CAD build for the part. Positions are in the model's coordinates, mm. A direction names the side the tool comes from. Coordinates: 2 decimals unless noted, no trailing zeros. Write each loop counter-clockwise with the first axis right and the second up, starting at its lowest first coordinate (ties: lowest second). Pieces come first, ordered by that corner, then holes.
```python
from build123d import *

# Parameters (mm, degrees)
SKETCH1_W              = 42
SKETCH1_H              = 5.9
SKETCH1_W_2            = 39.2
SKETCH1_H_2            = 3.95
BOSS_EXTRUDE1_DEPTH    = 32.25
FILLET2_R              = 3
SKETCH2_W              = 51.5
SKETCH2_H              = 13.6
SKETCH2_W_2            = 39.2
SKETCH2_H_2            = 3.95
BOSS_EXTRUDE2_DEPTH    = 5.8
SKETCH3_W              = 51.5
SKETCH3_H              = 13.6
SKETCH3_W_2            = 39.2
SKETCH3_H_2            = 3.95
BOSS_EXTRUDE3_DEPTH    = 5.8
SKETCH4_R              = 1.7
CUT_EXTRUDE1_DEPTH     = 62.792596644
SKETCH8_W              = 5.8
SKETCH8_H              = 7.5
BOSS_EXTRUDE4_DEPTH    = 13.6
M2_CLEARANCE_HOLE1_D   = 2.4
CUT_EXTRUDE4_DEPTH     = 4
SKETCH15_W             = 39.2
SKETCH15_H             = 3.95
CUT_EXTRUDE5_DEPTH     = 79.468767672
SKETCH17_R             = 2
CUT_EXTRUDE6_DEPTH     = 79.468767672
M3_CLEARANCE_HOLE1_D   = 3.4
CUT_EXTRUDE8_START     = -13.6
CUT_EXTRUDE8_OUTLINE_W = 5.8
CUT_EXTRUDE8_OUTLINE_H = 7.5
CUT_EXTRUDE8_OUTLINE_R = 1.7
CUT_EXTRUDE8_DEPTH     = 4.55
FILLET3_R              = 1


# Read off the part's stored shape, not the designer's step: Cut-Extrude8
with BuildPart() as part:
    # Sketch1 → Boss-Extrude1 (new body)
    with BuildSketch(Plane(origin=(0, 0, 0), x_dir=(0, 0, -1), z_dir=(1, 0, 0))):
        with Locations((21, 2.95)):
            Rectangle(SKETCH1_W, SKETCH1_H)
        with Locations((21, 2.95)):
            Rectangle(SKETCH1_W_2, SKETCH1_H_2, mode=Mode.SUBTRACT)
    extrude(amount=BOSS_EXTRUDE1_DEPTH)

    # Fillet2
    # the kernel refuses this fillet: 3 mm, written as the material it takes off along each edge
    with BuildSketch(Plane(origin=(-7.5, 0, -42), x_dir=(0, 0, 1), z_dir=(1, 0, 0)), Plane(origin=(-7.5, 5.9, 0), x_dir=(0, 0, -1), z_dir=(1, 0, 0)), Plane(origin=(-7.5, 5.9, -42), x_dir=(0, -1, 0), z_dir=(1, 0, 0))) as fillet2_piece_1:
        with BuildLine():
            CenterArc((FILLET2_R, -FILLET2_R), FILLET2_R, 90, 90)
            Line((0, -FILLET2_R), (0, 0))
            Line((0, 0), (FILLET2_R, 0))
        make_face()
    extrude(amount=47.25, mode=Mode.SUBTRACT)
    with BuildSketch(Plane(origin=(-7.5, 0, 0), x_dir=(0, 0, -1), z_dir=(1, 0, 0))) as fillet2_piece_2:
        with BuildLine():
            CenterArc((FILLET2_R, FILLET2_R), FILLET2_R, 180, 90)
            Line((0, FILLET2_R), (0, 0))
            Line((0, 0), (FILLET2_R, 0))
        make_face()
    extrude(amount=47.25, mode=Mode.SUBTRACT)

    # Sketch2 → Boss-Extrude2 (add)
    with BuildSketch(Plane(origin=(32.25, 0, 0), x_dir=(0, 0, -1), z_dir=(1, 0, 0))):
        with Locations((21, 2.95)):
            Rectangle(SKETCH2_W, SKETCH2_H)
        with Locations((21, 2.95)):
            Rectangle(SKETCH2_W_2, SKETCH2_H_2, mode=Mode.SUBTRACT)
    extrude(amount=BOSS_EXTRUDE2_DEPTH)

    # Sketch3 → Boss-Extrude3 (add)
    with BuildSketch(Plane.ZY):
        with Locations((-21, 2.95)):
            Rectangle(SKETCH3_W, SKETCH3_H)
        with Locations((-21, 2.95)):
            Rectangle(SKETCH3_W_2, SKETCH3_H_2, mode=Mode.SUBTRACT)
    extrude(amount=BOSS_EXTRUDE3_DEPTH)

    # Sketch4 → Cut-Extrude1 (cut, through all)
    with BuildSketch(Plane(origin=(0, 9.75, 0), x_dir=(1, 0, 0), z_dir=(0, 1, 0))):
        with Locations(Location((-2.9, 43.85, 0), (0, 0, 270))):
            Circle(SKETCH4_R)
        with Locations(Location((35.15, 43.85, 0), (0, 0, 270))):
            Circle(SKETCH4_R)
        with Locations(Location((-2.9, -1.85, 0), (0, 0, 270))):
            Circle(SKETCH4_R)
        with Locations(Location((35.15, -1.85, 0), (0, 0, 270))):
            Circle(SKETCH4_R)
    extrude(amount=-CUT_EXTRUDE1_DEPTH, mode=Mode.SUBTRACT)

    # Sketch8 → Boss-Extrude4 (add)
    with BuildSketch(Plane(origin=(0, 9.75, 0), x_dir=(1, 0, 0), z_dir=(0, 1, 0))):
        with Locations((-2.9, 50.5)):
            Rectangle(SKETCH8_W, SKETCH8_H)
        with Locations((-2.9, -8.5)):
            Rectangle(SKETCH8_W, SKETCH8_H)
        with BuildLine():
            Line((46.05, 25), (46.05, 49.75))
            Line((46.05, 49.75), (32.25, 49.75))
            Line((32.25, 49.75), (32.25, 46.75))
            Line((32.25, 46.75), (38.05, 46.75))
            Line((38.05, 46.75), (38.05, -4.75))
            Line((38.05, -4.75), (32.25, -4.75))
            Line((32.25, -4.75), (32.25, -7.75))
            Line((32.25, -7.75), (46.05, -7.75))
            Line((46.05, -7.75), (46.05, 17))
            ThreePointArc((46.05, 17), (50.05, 21), (46.05, 25))
        make_face()
    extrude(amount=-BOSS_EXTRUDE4_DEPTH)

    # M2 Clearance Hole1 (through all)
    with Locations(Plane(origin=(0, 9.75, 0), x_dir=(1, 0, 0), z_dir=(0, 1, 0))):
        with Locations((46.05, 21)):
            Hole(M2_CLEARANCE_HOLE1_D / 2)

    # Sketch14 → Cut-Extrude4 (cut)
    with BuildSketch(Plane.XZ.offset(3.85)):
        Polygon((43.625128869, -21), (44.837564435, -23.1), (47.262435565, -23.1), (48.474871131, -21), (47.262435565, -18.9), (44.837564435, -18.9), align=None)
    extrude(amount=-CUT_EXTRUDE4_DEPTH, mode=Mode.SUBTRACT)

    # Sketch15 → Cut-Extrude5 (cut, through all)
    with BuildSketch(Plane.ZY.offset(5.8)):
        with Locations((-21, 2.95)):
            Rectangle(SKETCH15_W, SKETCH15_H)
    extrude(amount=-CUT_EXTRUDE5_DEPTH, mode=Mode.SUBTRACT)

    # Sketch17 → Cut-Extrude6 (cut, through all)
    with BuildSketch(Plane.ZY.offset(5.8)):
        with Locations((-21, 2.95)):
            Circle(SKETCH17_R)
    extrude(amount=-CUT_EXTRUDE6_DEPTH, mode=Mode.SUBTRACT)

    # M3 Clearance Hole1 (through all)
    with Locations(Plane(origin=(-2.9, 9.75, -51.25), x_dir=(0, 0, 1), z_dir=(0, 1, 0))):
        with Locations((0, 0), (4.25, 44.1), (56.25, 44.1), (60.5, 0)):
            Hole(M3_CLEARANCE_HOLE1_D / 2)

    # Cut-Extrude8 outline → Cut-Extrude8 (cut)
    # profile 1 of 4: a face of its own
    with BuildSketch(Plane(origin=(0, 9.75, 0), x_dir=(1, 0, 0), z_dir=(0, 1, 0)).offset(CUT_EXTRUDE8_START)):
        with Locations((-2.9, 50.5)):
            Rectangle(CUT_EXTRUDE8_OUTLINE_W, CUT_EXTRUDE8_OUTLINE_H)
        with Locations((-2.9, 51.25)):
            Circle(CUT_EXTRUDE8_OUTLINE_R, mode=Mode.SUBTRACT)
    # profile 2 of 4: a face of its own
    with BuildSketch(Plane(origin=(0, 9.75, 0), x_dir=(1, 0, 0), z_dir=(0, 1, 0)).offset(CUT_EXTRUDE8_START)):
        with Locations((-2.9, -8.5)):
            Rectangle(CUT_EXTRUDE8_OUTLINE_W, CUT_EXTRUDE8_OUTLINE_H)
        with Locations((-2.9, -9.25)):
            Circle(CUT_EXTRUDE8_OUTLINE_R, mode=Mode.SUBTRACT)
    # profile 3 of 4: a face of its own
    with BuildSketch(Plane(origin=(0, 9.75, 0), x_dir=(1, 0, 0), z_dir=(0, 1, 0)).offset(CUT_EXTRUDE8_START)):
        Polygon((32.25, 49.75), (32.25, 46.75), (38.05, 46.75), (38.05, 41.7), (46.05, 41.7), (46.05, 49.75), align=None)
        with Locations((41.2, 47)):
            Circle(CUT_EXTRUDE8_OUTLINE_R, mode=Mode.SUBTRACT)
    # profile 4 of 4: a face of its own
    with BuildSketch(Plane(origin=(0, 9.75, 0), x_dir=(1, 0, 0), z_dir=(0, 1, 0)).offset(CUT_EXTRUDE8_START)):
        Polygon((38.05, -4.75), (32.25, -4.75), (32.25, -7.75), (46.05, -7.75), (46.05, 0.3), (38.05, 0.3), align=None)
        with Locations((41.2, -5)):
            Circle(CUT_EXTRUDE8_OUTLINE_R, mode=Mode.SUBTRACT)
    extrude(amount=CUT_EXTRUDE8_DEPTH, mode=Mode.SUBTRACT)

    # Fillet3
    fillet3_edges = [part.edges().sort_by_distance(p)[0] for p in [
        (46.05, -1.4375, -25),
        (46.05, -1.4375, -17),
        (46.05, 7.3375, -17),
        (46.05, 7.3375, -25),
        (39.15, 0.7, -49.75),
        (42.05, -3.85, -41.7),
        (38.05, -3.85, -44.225),
        (35.15, -3.85, -46.75),
        (38.05, 0.7, -44.225),
        (42.05, 0.7, -41.7),
        (38.05, -1.575, -41.7),
        (42.05, 0.7, -0.3),
        (35.15, -3.85, 4.75),
        (38.05, -3.85, 2.225),
        (39.15, 0.7, 7.75),
        (42.05, -3.85, -0.3),
        (38.05, 0.7, 2.225),
        (38.05, -1.575, -0.3),
        (-2.9, 0.7, 12.25),
        (-2.9, -3.85, 4.75),
        (-2.9, -3.85, -46.75),
        (-2.9, 0.7, -54.25),
    ]]
    fillet(fillet3_edges, radius=FILLET3_R)


solid = part.part
```
Item 1: Saw through at B-B, the plane z = -43.85. Write the cut outline in (x, y), and give its area (3 significant figures).
Item 2: Wall check: line 1 along X through (y, z) = (5.5, -43.85); line 2 along X through (y, z) = (7.1, -21); line 3 along X through (y, z) = (7.5, -4). Give the ranges that are in metal, low to high.
Item 3: Two-plate mould, pull along Y, no slides. Class faces 6 (the flat face through (20, 3, -40.6)), 7 (the flat face through (-3, 9.75, -21)), 8 (the flat face through (41, 0.7, -45)), 9 (the flat face through (46.05, 6, -4)): +Y half, -Y half, draft (parallel to the pull), parting line (faces both ways), or undercut.
Item 4: Which spindle directions (+Z, -Z, +X, -X, +Y, -Y) get a long thin tool onto all of the face, cutting with end or side? Do faces 1 (the flat face through (43, -2, -41.7)), 2 (the flat face through (46, -2, -18.9)), 3 (the flat face through (35, -1, 4.75)), 4 (the flat face through (23, 0.975, -11)), 5 (the flat face through (-3, 0.7, -49)). Say none if no direction does.
Item 5: Saw through at D-D, the plane z = -6.5. Write the cut outline in (x, y) (3 decimals).
Item 6: Saw through at A-A, the plane x = 41.2. State how many separate pieces and enclosed holes the cut face has, and give its area (3 significant figures).
Item 7: Flat gauge pins, fed straight in: pin 1 Ø6 at (x, y) = (37.5, 3) entering from +Z; pin 2 Ø2 at (x, y) = (33, -1) entering from -Z; pin 3 Ø1.8 at (x, y) = (34, -1) entering from +Z. Where does each tip first touch, or does it go through?
Working result:
1. outline: (-5.8, -3.85) - (-4.6, -3.85) - (-4.6, 9.75) - (-5.8, 9.75) - close; (-1.2, -3.85) - (0, -3.85) - (0, 9.75) - (-1.2, 9.75) - close; (32.25, -3.85) - (33.45, -3.85) - (33.45, 9.75) - (32.25, 9.75) - close; (36.85, -3.85) - (37.05, -3.85) arc R1 ccw to (38.05, -2.85) - (38.05, -0.3) arc R1 cw to (39.05, 0.7) - (46.05, 0.7) - (46.05, 9.75) - (36.85, 9.75) - close
1. area: 138 mm2
2. line 1: x = -5.8 to -4.6, -1.2 to 0, 32.25 to 33.45, 36.85 to 46.05
2. line 2: x = -5.8 to 0, 32.25 to 44.85, 47.25 to 50.05
2. line 3: x = -5.8 to 0, 32.25 to 46.05
3. face 6: undercut
3. face 7: +Y half
3. face 8: -Y half
3. face 9: draft
4. face 1: -Z, +X, -Y
4. face 2: -Y
4. face 3: +Z, +X, -X, -Y
4. face 4: +X, -X
4. face 5: -Z, +X, -X, -Y
5. outline: (-5.8, -3.85) - (0, -3.85) - (0, 0) - (32.25, 0) - (32.25, -3.85) - (46.05, -3.85) - (46.05, 0.975) - (-5.8, 0.975) - close; (-5.8, 4.925) - (46.05, 4.925) - (46.05, 9.75) - (32.25, 9.75) - (32.25, 5.9) - (0, 5.9) - (0, 9.75) - (-5.8, 9.75) - close
6. separate pieces: 3
6. enclosed holes: 1
6. area: 492 mm2
7. pin 1: stops at z = 7.75
7. pin 2: stops at z = -46.75
7. pin 3: stops at z = 4.75
